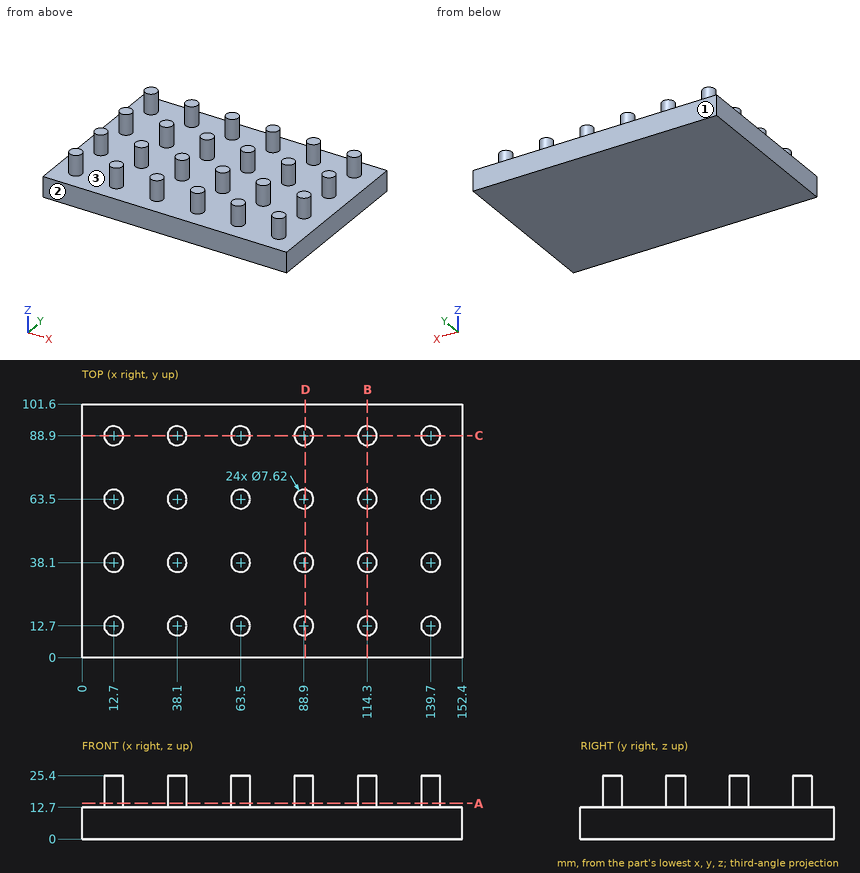
Design review of the part shown in the three views and the two pictorial views. Dimensions are in mm from the part's minimum x, y and z. Give positions to 0.01 mm unless a question says otherwise; leave off trailing zeros. Loops run counter-clockwise (first coordinate to the right, second up) from the corner with the lowest first, then second, coordinate; pieces in that order, holes last. Notation, with made-up numbers: (23, -16) -> (58, -16) arc R32 ccw to (58, 17) -> close; hole circle Ø7 at (24, 86). An arc over 180 degrees is marked (long way). Answer as a JSON object with one key per item and string values. Group by question number.
Q1. Take a section at C-C (y = 88.9). Write out the cut boundary in (x, z), plus the area to 3 significant figures.
Q2. Wall thickness on line 1 along Y through (x, z) = (63, 23.5); line 2 along Y through (x, z) = (16, 19.5); line 3 along X through (y, z) = (15, 14): over which ranges is each line inside the solid? List them lowest first.
Q3. Insertion check: pin 1 (3 mm diameter, centred on x = 45.5, y = 47, fed in from +Z); pin 2 (2 mm diameter, centred on x = 41, z = 17, fed in from +Y); pin 3 (6 mm diameter, centred on x = 67.5, z = 20.5, fed in from +Y). Each pin has a flat end and moves straight along its axis. Give the tip position at first contact, or say it passes through.
Q4. Take a section at D-D (x = 89.5). Write out the cut boundary in (y, z).
Q5. Take a section at A-A (z = 14.25). State how many separate pieces and enclosed holes the cut face has, plus the area to 3 significant figures.
Q6. Take a section at B-B (x = 114.3). Write out the cut boundary in (y, z), plus the area to 3 significant figures.
Q7. Draft analysis for pull direction Y (two halves, no side actions). For the marked faces 1, 2 and 3, state which applies: pulls with the +Y half, pulls with the -Y half, needs draft (parallel to the pull), parting line crosses it, or undercut.
Answer below:
{
 "1": {"outline": "(0, 0) -> (152.4, 0) -> (152.4, 12.7) -> (143.51, 12.7) -> (143.51, 25.4) -> (135.89, 25.4) -> (135.89, 12.7) -> (118.11, 12.7) -> (118.11, 25.4) -> (110.49, 25.4) -> (110.49, 12.7) -> (92.71, 12.7) -> (92.71, 25.4) -> (85.09, 25.4) -> (85.09, 12.7) -> (67.31, 12.7) -> (67.31, 25.4) -> (59.69, 25.4) -> (59.69, 12.7) -> (41.91, 12.7) -> (41.91, 25.4) -> (34.29, 25.4) -> (34.29, 12.7) -> (16.51, 12.7) -> (16.51, 25.4) -> (8.89, 25.4) -> (8.89, 12.7) -> (0, 12.7) -> close", "area": "2,520 mm2"},
 "2": {"line 1": "y = 8.92 to 16.48, 34.32 to 41.88, 59.72 to 67.28, 85.12 to 92.68", "line 2": "y = 10.8 to 14.6, 36.2 to 40, 61.6 to 65.4, 87 to 90.8", "line 3": "x = 9.66 to 15.74, 35.06 to 41.14, 60.46 to 66.54, 85.86 to 91.94, 111.26 to 117.34, 136.66 to 142.74"},
 "3": {"pin 1": "stops at z = 12.7", "pin 2": "stops at y = 92.2", "pin 3": "stops at y = 92.58"},
 "4": {"outline": "(0, 0) -> (101.6, 0) -> (101.6, 12.7) -> (92.66, 12.7) -> (92.66, 25.4) -> (85.14, 25.4) -> (85.14, 12.7) -> (67.26, 12.7) -> (67.26, 25.4) -> (59.74, 25.4) -> (59.74, 12.7) -> (41.86, 12.7) -> (41.86, 25.4) -> (34.34, 25.4) -> (34.34, 12.7) -> (16.46, 12.7) -> (16.46, 25.4) -> (8.94, 25.4) -> (8.94, 12.7) -> (0, 12.7) -> close"},
 "5": {"separate pieces": "24", "enclosed holes": "0", "area": "1,090 mm2"},
 "6": {"outline": "(0, 0) -> (101.6, 0) -> (101.6, 12.7) -> (92.71, 12.7) -> (92.71, 25.4) -> (85.09, 25.4) -> (85.09, 12.7) -> (67.31, 12.7) -> (67.31, 25.4) -> (59.69, 25.4) -> (59.69, 12.7) -> (41.91, 12.7) -> (41.91, 25.4) -> (34.29, 25.4) -> (34.29, 12.7) -> (16.51, 12.7) -> (16.51, 25.4) -> (8.89, 25.4) -> (8.89, 12.7) -> (0, 12.7) -> close", "area": "1,680 mm2"},
 "7": {"face 1": "pulls with the +Y half", "face 2": "pulls with the -Y half", "face 3": "undercut"}
}
